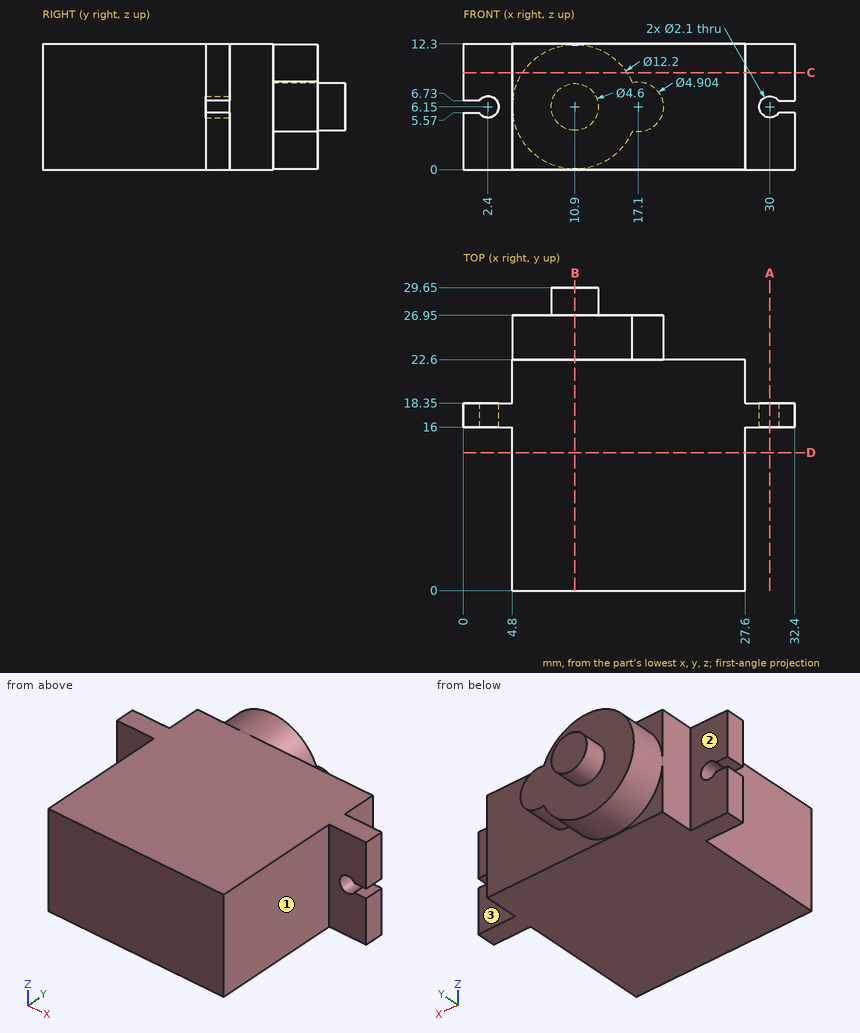
Source: three-view drawing plus pictorial views. Frame: mm from the lowest corner of the part. A direction names the side the tool comes from. Round coordinates to 2 decimals unless told otherwise and drop trailing zeros. Write each loop counter-clockwise with the first axis right and the second up, starting at its lowest first coordinate (ties: lowest second). Pieces come first, ordered by that corner, then holes. Notation, with made-up numbers: M -20.5,48 L -11.5,48 A37 ccw -11.5,85 Z; hole C 89.25,8.5 d2. An arc over 180 degrees is marked long. One line per item, written item: value. Start each with the question number.
Item 1: Section query A-A (x = 30). Return the cut outline in (y, z), plus the area to 3 significant figures.
Item 2: Set-up query: the marked faces 1, 2 and 3. Return all of +Z, -Z, +X, -X, +Y, -Y with unobstructed straight access to the full face (end or side cutting, diameter ignored); none if empty.
Item 3: Section query C-C (z = 9.5). Return the cut outline in (x, y), plus the area to 3 significant figures.
Item 4: Section query D-D (y = 13.5). Return the cut outline in (x, z), plus the area to 3 significant figures.
Item 5: Ray query, L1, parallel to Z at x = 30, y = 17.85; L2, parallel to X at y = 22.5, z = 7.75; L3, parallel to Y at x = 25.5, z = 6. Return the intervals inside material, ascending. Write a range as from..to.
Item 6: Pin query (flat end, axial travel): pin 1 (2 mm diameter, centred on y = 20.5, z = 6.5, fed in from +X); pin 2 (2.5 mm diameter, centred on x = 29, z = 5.5, fed in from +Y); pin 3 (1.3 mm diameter, centred on y = 20.5, z = 6, fed in from -X). Return the tip coordinate at first contact, or that it passes through.
Item 7: Section query B-B (x = 10.9). Return the cut outline in (y, z), plus the area to 3 significant figures.
Result set:
1. outline: M 16,0 L 18.35,0 L 18.35,5.1 L 16,5.1 Z; M 16,7.2 L 18.35,7.2 L 18.35,12.3 L 16,12.3 Z
1. area: 24.0 mm²
2. face 1: +Z, -Z, +X, -Y
2. face 2: +Z, -Z, -X, +Y
2. face 3: +Z, -Z, +X, +Y
3. outline: M 0,16 L 4.8,16 L 4.8,0 L 27.6,0 L 27.6,16 L 32.4,16 L 32.4,18.35 L 27.6,18.35 L 27.6,22.6 L 16,22.6 L 16,26.95 L 5.8,26.95 L 5.8,22.6 L 4.8,22.6 L 4.8,18.35 L 0,18.35 Z
3. area: 582 mm²
4. outline: M 4.8,0 L 27.6,0 L 27.6,12.3 L 4.8,12.3 Z
4. area: 280 mm²
5. L1: z = 0..5.1, 7.2..12.3
5. L2: x = 4.8..27.6
5. L3: y = 0..22.6
6. pin 1: stops at x = 27.6
6. pin 2: stops at y = 18.35
6. pin 3: stops at x = 4.8
7. outline: M 0,0 L 22.6,0 L 22.6,0.05 L 26.95,0.05 L 26.95,3.85 L 29.65,3.85 L 29.65,8.45 L 26.95,8.45 L 26.95,12.25 L 22.6,12.25 L 22.6,12.3 L 0,12.3 Z
7. area: 343 mm²
